Geometry check sheet. Reference: the model listing, model coordinates, mm. A direction names the side the tool comes from. Give positions to 0.01 mm unless a question says otherwise; leave off trailing zeros. Write each loop counter-clockwise with the first axis right and the second up, starting at its lowest first coordinate (ties: lowest second). Pieces come first, ordered by that corner, then holes. Notation, with made-up numbers: (53, -23) - (76, -23) arc R20 ccw to (76, -2) - close; hole circle Ø8 at (-16.75, 49.25). An arc over 180 degrees is marked (long way). Use a Markdown table: item, result.
```python
from build123d import *

# Parameters (mm, degrees)
SKETCH1_W                        = 45
SKETCH1_H                        = 40
CONNECTION_BASE_DEPTH            = 5
SKETCH9_R                        = 3.2
SKETCH9_R_2                      = 1.6
LEFT_LEG_DEPTH                   = 5
LEG_FILLET_R                     = 5
HUB_FILLET_R                     = 10
LEG_FILLET_OF_MIRROR_RIGHT_LEG_R = 5
HUB_FILLET_OF_MIRROR_RIGHT_LEG_R = 10
SKETCH2_R                        = 2
BASE_CONN_HOLE_DEPTH             = 94.482952991
BASE_CONN_NUT_DEPTH              = 2
BASE_HOLES_PATTERN_COUNT         = 2
BASE_HOLES_PATTERN_PITCH         = 20
BASE_HOLES_PATTERN_COUNT_DIR2    = 2
BASE_HOLES_PATTERN_PITCH_DIR2    = 20
SKETCH4_W                        = 55
SKETCH4_H                        = 4
MOTOR_STEP_DEPTH                 = 6.16
SKETCH5_W                        = 55
SKETCH5_H                        = 22
MOTOR_SHELF_DEPTH                = 5
MOTOR_M3_5X0_6_TAPPED_HOLE1_D    = 2.9
SMALL_INTERNAL_FILLETS_R         = 1


# Some blends are built 0.0001 mm under size
with BuildPart() as part:
    # Sketch1 → Connection_Base (new body)
    with BuildSketch(Plane(origin=(0, 0, 0), x_dir=(1, 0, 0), z_dir=(0, 1, 0))):
        with Locations((-2.5, 0)):
            Rectangle(SKETCH1_W, SKETCH1_H)
    extrude(amount=CONNECTION_BASE_DEPTH)

    # Sketch9 → LEFT_LEG (add)
    with BuildSketch(Plane.XY.offset(10)):
        with BuildLine():
            Line((-51.756098166, 5), (-73, 5))
            Line((-73, 5), (-73, 10))
            ThreePointArc((-73, 10), (-80, 17), (-87, 10))
            Line((-87, 10), (-87, 0))
            Line((-87, 0), (0, 0))
            Line((0, 0), (0, 5))
            Line((0, 5), (-46.756098166, 5))
            Line((-46.756098166, 5), (-46.756098166, 23.419872981))
            ThreePointArc((-46.756098166, 23.419872981), (-49.256098166, 32.75), (-51.756098166, 23.419872981))
            Line((-51.756098166, 23.419872981), (-51.756098166, 5))
        make_face()
        with Locations((-80, 10)):
            Circle(SKETCH9_R, mode=Mode.SUBTRACT)
        with Locations((-49.256098166, 27.75)):
            Circle(SKETCH9_R_2, mode=Mode.SUBTRACT)
    left_leg = extrude(amount=LEFT_LEG_DEPTH)

    # LEG_Fillet
    leg_fillet_edges = [part.edges().sort_by_distance(p)[0] for p in [
        (-51.756098166, 5, 12.5),
        (-46.756098166, 5, 12.5),
        (-73, 5, 12.5),
    ]]
    fillet(leg_fillet_edges, radius=LEG_FILLET_R - 0.0001)  # a hair under: the kernel refuses the full size

    # Hub_Fillet
    hub_fillet_edges = [part.edges().sort_by_distance(p)[0] for p in [
        (-46.756098166, 23.419872981, 12.5),
        (-51.756098166, 23.419872981, 12.5),
    ]]
    fillet(hub_fillet_edges, radius=HUB_FILLET_R)

    # Mirror_RIGHT_LEG: LEFT_LEG across plane
    add(left_leg.mirror(Plane.XY))

    # LEG_Fillet of Mirror_RIGHT_LEG
    leg_fillet_of_mirror_right_leg_edges = [part.edges().sort_by_distance(p)[0] for p in [
        (-51.756098166, 5, -12.5),
        (-46.756098166, 5, -12.5),
        (-73, 5, -12.5),
    ]]
    fillet(leg_fillet_of_mirror_right_leg_edges, radius=LEG_FILLET_OF_MIRROR_RIGHT_LEG_R - 0.0001)  # a hair under: the kernel refuses the full size

    # Hub_Fillet of Mirror_RIGHT_LEG
    hub_fillet_of_mirror_right_leg_edges = [part.edges().sort_by_distance(p)[0] for p in [
        (-46.756098166, 23.419872981, -12.5),
        (-51.756098166, 23.419872981, -12.5),
    ]]
    fillet(hub_fillet_of_mirror_right_leg_edges, radius=HUB_FILLET_OF_MIRROR_RIGHT_LEG_R)

    # Sketch2 → Base_Conn_Hole (cut, through all)
    with BuildSketch(Plane(origin=(0, 5, 0), x_dir=(1, 0, 0), z_dir=(0, 1, 0))):
        with Locations(Location((-10, 10, 0), (0, 0, 270))):
            Circle(SKETCH2_R)
    base_conn_hole = extrude(amount=-BASE_CONN_HOLE_DEPTH, mode=Mode.SUBTRACT)

    # Sketch3 → Base_Conn_Nut (cut)
    with BuildSketch(Plane(origin=(0, 5, 0), x_dir=(1, 0, 0), z_dir=(0, 1, 0))):
        Polygon((-7.979274058, 6.5), (-5.958548116, 10), (-7.979274058, 13.5), (-12.020725942, 13.5), (-14.041451884, 10), (-12.020725942, 6.5), align=None)
    base_conn_nut = extrude(amount=-BASE_CONN_NUT_DEPTH, mode=Mode.SUBTRACT)

    # Base_Holes_Pattern: Base_Conn_Hole, Base_Conn_Nut 2 × 2
    with Locations(*[(j * BASE_HOLES_PATTERN_PITCH_DIR2, 0, i * BASE_HOLES_PATTERN_PITCH) for i in range(BASE_HOLES_PATTERN_COUNT) for j in range(BASE_HOLES_PATTERN_COUNT_DIR2) if (i, j) != (0, 0)]):
        add(base_conn_hole, mode=Mode.SUBTRACT)
        add(base_conn_nut, mode=Mode.SUBTRACT)

    # Sketch4 → Motor_Step (add)
    with BuildSketch(Plane(origin=(0, 5, 0), x_dir=(1, 0, 0), z_dir=(0, 1, 0))):
        with Locations((-17.5, 16)):
            Rectangle(SKETCH4_W, SKETCH4_H)
    extrude(amount=MOTOR_STEP_DEPTH)

    # Sketch5 → Motor_Shelf (add)
    with BuildSketch(Plane(origin=(0, 11.16, 0), x_dir=(1, 0, 0), z_dir=(0, 1, 0))):
        with Locations((-17.5, 25)):
            Rectangle(SKETCH5_W, SKETCH5_H)
    extrude(amount=MOTOR_SHELF_DEPTH)

    # Motor_M3.5x0.6 Tapped Hole1 (through all)
    with Locations(Plane(origin=(0, 16.16, 0), x_dir=(1, 0, 0), z_dir=(0, 1, 0))):
        with Locations((3, 21), (3, 33), (-40, 33), (-40, 21)):
            Hole(MOTOR_M3_5X0_6_TAPPED_HOLE1_D / 2)

    # Small_Internal_Fillets
    # the kernel refuses this fillet: 1 mm, written as the material it adds along each edge
    with BuildSketch(Plane(origin=(-25, 0, 10), x_dir=(0, 0, -1), z_dir=(0, 1, 0)), Plane(origin=(-25, 0, 15), x_dir=(-1, 0, 0), z_dir=(0, 1, 0)), Plane(origin=(-25, 0, -10), x_dir=(-1, 0, 0), z_dir=(0, 1, 0))) as small_internal_fillets_piece_1:
        with BuildLine():
            CenterArc((SMALL_INTERNAL_FILLETS_R, SMALL_INTERNAL_FILLETS_R), SMALL_INTERNAL_FILLETS_R, 180, 90)
            Line((0, SMALL_INTERNAL_FILLETS_R), (0, 0))
            Line((0, 0), (SMALL_INTERNAL_FILLETS_R, 0))
        make_face()
    extrude(amount=5)
    with BuildSketch(Plane(origin=(-41.756198166, 9.9999, -14), x_dir=(0, -1, 0), z_dir=(1, 0, 0))) as small_internal_fillets_piece_2_section:
        with BuildLine():
            CenterArc((4.9999 - SMALL_INTERNAL_FILLETS_R, -SMALL_INTERNAL_FILLETS_R), SMALL_INTERNAL_FILLETS_R, 0, 90)
            Line((4.9999 - SMALL_INTERNAL_FILLETS_R, 0), (4.9999, 0))
            Line((4.9999, 0), (4.9999, -SMALL_INTERNAL_FILLETS_R))
        make_face()
    small_internal_fillets_piece_2 = revolve(axis=Axis((-41.756198166, 9.9999, -14), (0, 0, -1)), revolution_arc=69.099967659, mode=Mode.PRIVATE)
    small_internal_fillets_piece_2 = split(small_internal_fillets_piece_2, bisect_by=Plane(origin=(-45, 9.9999, -14), z_dir=(1, 0, 0)), keep=Keep.TOP, mode=Mode.PRIVATE)
    add(small_internal_fillets_piece_2)
    with BuildSketch(Plane(origin=(10, 5, -14), x_dir=(0, 0, 1), z_dir=(-1, 0, 0))) as small_internal_fillets_piece_3_section:
        with BuildLine():
            CenterArc((SMALL_INTERNAL_FILLETS_R, SMALL_INTERNAL_FILLETS_R), SMALL_INTERNAL_FILLETS_R, 180, 90)
            Line((0, SMALL_INTERNAL_FILLETS_R), (0, 0))
            Line((0, 0), (SMALL_INTERNAL_FILLETS_R, 0))
        make_face()
    small_internal_fillets_piece_3 = extrude(amount=51.756198166, mode=Mode.PRIVATE)
    small_internal_fillets_piece_3 = split(small_internal_fillets_piece_3, bisect_by=Plane(origin=(10, 5, -13.5), z_dir=(0, 0, -1)), keep=Keep.TOP, mode=Mode.PRIVATE)
    add(small_internal_fillets_piece_3)
    with BuildSketch(Plane(origin=(12.5, 5, -14), x_dir=(0, 0, 1), z_dir=(-1, 0, 0))) as small_internal_fillets_piece_4_section:
        with BuildLine():
            CenterArc((SMALL_INTERNAL_FILLETS_R, SMALL_INTERNAL_FILLETS_R), SMALL_INTERNAL_FILLETS_R, 180, 90)
            Line((0, SMALL_INTERNAL_FILLETS_R), (0, 0))
            Line((0, 0), (SMALL_INTERNAL_FILLETS_R, 0))
        make_face()
    small_internal_fillets_piece_4 = extrude(amount=54.256198166, mode=Mode.PRIVATE)
    small_internal_fillets_piece_4 = split(small_internal_fillets_piece_4, bisect_by=Plane(origin=(9.325961894, 5, -15.832531755), z_dir=(-0.8660254037844387, 0, -0.4999999999999999)), keep=Keep.TOP, mode=Mode.PRIVATE)
    small_internal_fillets_piece_4 = split(small_internal_fillets_piece_4, bisect_by=Plane(origin=(-3.075961894, 5, -5.007214207), z_dir=(0.8660254037844389, 0, -0.4999999999999996)), keep=Keep.TOP, mode=Mode.PRIVATE)
    add(small_internal_fillets_piece_4)
    with BuildSketch(Plane(origin=(12.5, 5, -14), x_dir=(0, 0, 1), z_dir=(-1, 0, 0))) as small_internal_fillets_piece_5_section:
        with BuildLine():
            CenterArc((SMALL_INTERNAL_FILLETS_R, SMALL_INTERNAL_FILLETS_R), SMALL_INTERNAL_FILLETS_R, 180, 90)
            Line((0, SMALL_INTERNAL_FILLETS_R), (0, 0))
            Line((0, 0), (SMALL_INTERNAL_FILLETS_R, 0))
        make_face()
    small_internal_fillets_piece_5 = extrude(amount=54.256198166, mode=Mode.PRIVATE)
    small_internal_fillets_piece_5 = split(small_internal_fillets_piece_5, bisect_by=Plane(origin=(-5.674038106, 5, -24.492785793), z_dir=(-0.8660254037844387, 0, -0.4999999999999999)), keep=Keep.TOP, mode=Mode.PRIVATE)
    add(small_internal_fillets_piece_5)
    with BuildSketch(Plane(origin=(10, 5, -18), x_dir=(1, 0, 0), z_dir=(0, 0, 1))) as small_internal_fillets_piece_6:
        with BuildLine():
            CenterArc((SMALL_INTERNAL_FILLETS_R, SMALL_INTERNAL_FILLETS_R), SMALL_INTERNAL_FILLETS_R, 180, 90)
            Line((0, SMALL_INTERNAL_FILLETS_R), (0, 0))
            Line((0, 0), (SMALL_INTERNAL_FILLETS_R, 0))
        make_face()
    extrude(amount=4)
    with BuildSketch(Plane(origin=(-25, 5, -18), x_dir=(0, 0, -1), z_dir=(1, 0, 0))) as small_internal_fillets_piece_7:
        with BuildLine():
            CenterArc((SMALL_INTERNAL_FILLETS_R, SMALL_INTERNAL_FILLETS_R), SMALL_INTERNAL_FILLETS_R, 180, 90)
            Line((0, SMALL_INTERNAL_FILLETS_R), (0, 0))
            Line((0, 0), (SMALL_INTERNAL_FILLETS_R, 0))
        make_face()
    extrude(amount=35)
    with BuildSketch(Plane(origin=(-45, 11.16, -18), x_dir=(0, -1, 0), z_dir=(1, 0, 0))) as small_internal_fillets_piece_8:
        with BuildLine():
            CenterArc((SMALL_INTERNAL_FILLETS_R, SMALL_INTERNAL_FILLETS_R), SMALL_INTERNAL_FILLETS_R, 180, 90)
            Line((0, SMALL_INTERNAL_FILLETS_R), (0, 0))
            Line((0, 0), (SMALL_INTERNAL_FILLETS_R, 0))
        make_face()
    extrude(amount=55)
    with BuildSketch(Plane(origin=(10, 5, -18), x_dir=(1, 0, 0), z_dir=(0, 0, 1))) as small_internal_fillets_piece_9a_section:
        with BuildLine():
            CenterArc((SMALL_INTERNAL_FILLETS_R, SMALL_INTERNAL_FILLETS_R), SMALL_INTERNAL_FILLETS_R, 180, 90)
            Line((0, SMALL_INTERNAL_FILLETS_R), (0, 0))
            Line((0, 0), (SMALL_INTERNAL_FILLETS_R, 0))
        make_face()
    small_internal_fillets_piece_9a = extrude(amount=6.5, mode=Mode.PRIVATE)
    small_internal_fillets_piece_9a = split(small_internal_fillets_piece_9a, bisect_by=Plane(origin=(10, 5, -14), z_dir=(0, 0, 1)), keep=Keep.TOP, mode=Mode.PRIVATE)
    small_internal_fillets_piece_9a = split(small_internal_fillets_piece_9a, bisect_by=Plane(origin=(10, 5, -13.5), z_dir=(0, 0, -1)), keep=Keep.TOP, mode=Mode.PRIVATE)
    with BuildSketch(Plane(origin=(12.5, 5, -14), x_dir=(0, 0, 1), z_dir=(-1, 0, 0))) as small_internal_fillets_piece_9b_section:
        with BuildLine():
            CenterArc((SMALL_INTERNAL_FILLETS_R, SMALL_INTERNAL_FILLETS_R), SMALL_INTERNAL_FILLETS_R, 180, 90)
            Line((0, SMALL_INTERNAL_FILLETS_R), (0, 0))
            Line((0, 0), (SMALL_INTERNAL_FILLETS_R, 0))
        make_face()
    small_internal_fillets_piece_9b = extrude(amount=54.256198166, mode=Mode.PRIVATE)
    small_internal_fillets_piece_9b = split(small_internal_fillets_piece_9b, bisect_by=Plane(origin=(10, 5, -14), z_dir=(1, 0, 0)), keep=Keep.TOP, mode=Mode.PRIVATE)
    small_internal_fillets_piece_9b = split(small_internal_fillets_piece_9b, bisect_by=Plane(origin=(11.924038106, 5, -13.667468245), z_dir=(-0.8660254037844389, 0, 0.4999999999999996)), keep=Keep.TOP, mode=Mode.PRIVATE)
    small_internal_fillets_piece_9b = split(small_internal_fillets_piece_9b, bisect_by=Plane(origin=(12.5, 5, -13.5), z_dir=(0, 0, -1)), keep=Keep.TOP, mode=Mode.PRIVATE)
    small_internal_fillets_piece_9 = small_internal_fillets_piece_9a & small_internal_fillets_piece_9b
    add(small_internal_fillets_piece_9)
    with BuildSketch(Plane(origin=(-25, 5, -18), x_dir=(0, 0, -1), z_dir=(1, 0, 0))) as small_internal_fillets_piece_10a_section:
        with BuildLine():
            CenterArc((SMALL_INTERNAL_FILLETS_R, SMALL_INTERNAL_FILLETS_R), SMALL_INTERNAL_FILLETS_R, 180, 90)
            Line((0, SMALL_INTERNAL_FILLETS_R), (0, 0))
            Line((0, 0), (SMALL_INTERNAL_FILLETS_R, 0))
        make_face()
    small_internal_fillets_piece_10a = extrude(amount=37.5, mode=Mode.PRIVATE)
    small_internal_fillets_piece_10a = split(small_internal_fillets_piece_10a, bisect_by=Plane(origin=(10, 5, -18), z_dir=(1, 0, 0)), keep=Keep.TOP, mode=Mode.PRIVATE)
    with BuildSketch(Plane(origin=(10, 5, -20.5), x_dir=(1, 0, 0), z_dir=(0, 0, 1))) as small_internal_fillets_piece_10b_section:
        with BuildLine():
            CenterArc((SMALL_INTERNAL_FILLETS_R, SMALL_INTERNAL_FILLETS_R), SMALL_INTERNAL_FILLETS_R, 180, 90)
            Line((0, SMALL_INTERNAL_FILLETS_R), (0, 0))
            Line((0, 0), (SMALL_INTERNAL_FILLETS_R, 0))
        make_face()
    small_internal_fillets_piece_10b = extrude(amount=6.5, mode=Mode.PRIVATE)
    small_internal_fillets_piece_10b = split(small_internal_fillets_piece_10b, bisect_by=Plane(origin=(10, 5, -20), z_dir=(0, 0, 1)), keep=Keep.TOP, mode=Mode.PRIVATE)
    small_internal_fillets_piece_10b = split(small_internal_fillets_piece_10b, bisect_by=Plane(origin=(10, 5, -18), z_dir=(0, 0, -1)), keep=Keep.TOP, mode=Mode.PRIVATE)
    small_internal_fillets_piece_10 = small_internal_fillets_piece_10a & small_internal_fillets_piece_10b
    add(small_internal_fillets_piece_10)


solid = part.part
```
1) Set-up check for faces 1 (the flat face through (-13.045, 4.014, 11.726)), 2 (the cylindrical face through (-71, 6, -13)), 3 (the flat face through (-3, 2, 20)): record each of +Z, -Z, +X, -X, +Y, -Y from which the full face is reachable in a straight line by a thin tool's end or side.
Working result:
| item | result |
|---|---|
| face 1 | +Y |
| face 2 | +Z, -Z, +Y |
| face 3 | +Z, +X, -X, +Y, -Y |
2) Section check B-B on x = 3. Record the boundary of the cut face in (y, z).
Working result:
| item | result |
|---|---|
| outline | (0, -19.55) - (5, -19.55) - (5, -19) arc R1 cw to (6, -18) - (10.16, -18) arc R1 cw to (11.16, -19) - (11.16, -19.55) - (16.16, -19.55) - (16.16, -14) - (6, -14) arc R1 cw to (5, -13) - (5, 20) - (0, 20) - close; (11.16, -36) - (16.16, -36) - (16.16, -34.45) - (11.16, -34.45) - close; (11.16, -31.55) - (16.16, -31.55) - (16.16, -22.45) - (11.16, -22.45) - close |
3) Section check C-C on y = 14.5. Count the separate pieces of the cut face and the enclosed holes in it, then the cut area to 3 significant figures.
Working result:
| item | result |
|---|---|
| separate pieces | 5 |
| enclosed holes | 4 |
| area | 1,340 mm² |
4) Depth check by flat-ended pin: P1, Ø1, axis at x = -26, y = 14.5, coming from the +Z side; P2, Ø4, axis at x = -12.5, y = 8.5, coming from the -Z side; P3, Ø5, axis at x = -74, y = 15.5, coming from the -Z side. Enter the tip coordinate at first touch or a pass-through.
Working result:
| item | result |
|---|---|
| P1 | stops at z = -14 |
| P2 | stops at z = -18.06 |
| P3 | stops at z = -15 |
5) Mould release check, pull along X, two halves, no side actions. Record for faces 4 (the flat face through (-35, 5, -17)), 5 (the flat face through (-87, 5, -12)), 6 (the cylindrical face through (-48.4, 29.1, 12.5)): pulls with the +X half, pulls with the -X half, needs draft (parallel to the pull), parting line crosses it, or undercut.
Working result:
| item | result |
|---|---|
| face 4 | needs draft |
| face 5 | pulls with the -X half |
| face 6 | undercut |
6) Section check A-A on z = -33. Record the boundary of the cut face in (x, y), then the cut area to 3 significant figures.
Working result:
| item | result |
|---|---|
| outline | (-45, 11.16) - (-41.45, 11.16) - (-41.45, 16.16) - (-45, 16.16) - close; (-38.55, 11.16) - (1.55, 11.16) - (1.55, 16.16) - (-38.55, 16.16) - close; (4.45, 11.16) - (10, 11.16) - (10, 16.16) - (4.45, 16.16) - close |
| area | 246 mm² |
7) Section check D-D on y = 27.75. Record the boundary of the cut face in (x, z), then the cut area to 3 significant figures.
Working result:
| item | result |
|---|---|
| outline | (-54.26, -15) - (-50.86, -15) - (-50.86, -10) - (-54.26, -10) - close; (-54.26, 10) - (-50.86, 10) - (-50.86, 15) - (-54.26, 15) - close; (-47.66, -15) - (-44.26, -15) - (-44.26, -10) - (-47.66, -10) - close; (-47.66, 10) - (-44.26, 10) - (-44.26, 15) - (-47.66, 15) - close |
| area | 68.0 mm² |
8) Material ranges on L1, parallel to X at y = 14.2, z = -33; L2, parallel to Z at x = 3, y = 13; L3, parallel to Y at x = -80, z = 11, recorded low to high. Write a range as from..to.
Working result:
| item | result |
|---|---|
| L1 | x = -45..-41.45, -38.55..1.55, 4.45..10 |
| L2 | z = -36..-34.45, -31.55..-22.45, -19.55..-14 |
| L3 | y = 0..6.8, 13.2..17 |
